```python
from build123d import *

# Parameters (mm, degrees)
EXTRUDE_1_DEPTH       = 244
EXTRUDE_3_DEPTH       = 244
PATTERN_CURVE_1_COUNT = 19
PATTERN_CURVE_1_PITCH = 9.75
SKETCH_3_R            = 2.25
CUT_EXTRUDE_1_DEPTH   = 50
CUT_EXTRUDE_3_DEPTH   = 80
SKETCH_8_R            = 1.6
SKETCH_8_R_2          = 1.3
CUT_EXTRUDE_4_DEPTH   = 10
SKETCH_10_R           = 2.6
SKETCH_10_R_2         = 1.6
CUT_EXTRUDE_5_DEPTH   = 6
SKETCH_12_R           = 2.1
SKETCH_12_R_2         = 1.6
CUT_EXTRUDE_6_DEPTH   = 10


with BuildPart() as part:
    # Эскиз1 → Вытянуть1 (new body)
    with BuildSketch(Plane.XY):
        with BuildLine():
            Line((0, 45), (2.564446908, 45))
            ThreePointArc((2.564446908, 45), (3.247630994, 44.730246195), (3.562232066, 44.066519011))
            Line((3.562232066, 44.066519011), (5.5, 15))
            Line((5.5, 15), (194.5, 15))
            Line((194.5, 15), (196.437767934, 44.066519011))
            ThreePointArc((196.437767934, 44.066519011), (196.752369006, 44.730246195), (197.435553092, 45))
            Line((197.435553092, 45), (200, 45))
            Line((200, 45), (200, 0))
            Line((200, 0), (0, 0))
            Line((0, 0), (0, 45))
        make_face()
    extrude(amount=EXTRUDE_1_DEPTH)

    # Эскиз2 → Вытянуть3 (add)
    with BuildSketch(Plane.XY.offset(244)):
        with BuildLine():
            Line((11.5, 44.5), (10, 15))
            Line((10, 15), (14, 15))
            Line((14, 15), (12.5, 44.5))
            ThreePointArc((12.5, 44.5), (12, 45), (11.5, 44.5))
        make_face()
    extrude_3 = extrude(amount=-EXTRUDE_3_DEPTH)

    # Кривая1: Вытянуть3 ×19
    with Locations(*[(i * PATTERN_CURVE_1_PITCH, 0, 0) for i in range(1, PATTERN_CURVE_1_COUNT)]):
        add(extrude_3)

    # Эскиз3 → Вырез-Вытянуть1 (cut)
    with BuildSketch(Plane.XZ):
        with Locations((4, 236)):
            Circle(SKETCH_3_R)
        with Locations((74, 236)):
            Circle(SKETCH_3_R)
        with Locations(Location((74, 8, 0), (0, 0, 131.810314896))):
            Circle(SKETCH_3_R)
        with Locations(Location((4, 8, 0), (0, 0, 311.810314896))):
            Circle(SKETCH_3_R)
        with Locations((196, 8)):
            Circle(SKETCH_3_R)
        with Locations((126, 8)):
            Circle(SKETCH_3_R)
        with Locations(Location((126, 236, 0), (0, 0, 63.612200039))):
            Circle(SKETCH_3_R)
        with Locations(Location((196, 236, 0), (0, 0, 309.644601439))):
            Circle(SKETCH_3_R)
    extrude(amount=-CUT_EXTRUDE_1_DEPTH, mode=Mode.SUBTRACT)

    # Эскиз6 → Вырез-Вытянуть3 (cut)
    with BuildSketch(Plane.XZ.offset(-6)):
        with BuildLine():
            Line((9, 236), (9, 247.625328498))
            Line((9, 247.625328498), (-6.127764857, 247.625328498))
            Line((-6.127764857, 247.625328498), (-6.127764857, 231))
            Line((-6.127764857, 231), (4, 231))
            ThreePointArc((4, 231), (7.535533906, 232.464466094), (9, 236))
        make_face()
        with BuildLine():
            Line((69, 236), (69, 248.983105869))
            Line((69, 248.983105869), (79, 248.983105869))
            Line((79, 248.983105869), (79, 236))
            ThreePointArc((79, 236), (74, 231), (69, 236))
        make_face()
        with BuildLine():
            Line((121, 248.983105869), (121, 236))
            ThreePointArc((121, 236), (126, 231), (131, 236))
            Line((131, 236), (131, 248.983105869))
            Line((131, 248.983105869), (121, 248.983105869))
        make_face()
        with BuildLine():
            Line((206.127764857, 247.625328498), (191, 247.625328498))
            Line((191, 247.625328498), (191, 236))
            ThreePointArc((191, 236), (192.464466094, 232.464466094), (196, 231))
            Line((196, 231), (206.127764857, 231))
            Line((206.127764857, 231), (206.127764857, 247.625328498))
        make_face()
        with BuildLine():
            Line((191, 8), (191, -3.625328498))
            Line((191, -3.625328498), (206.127764857, -3.625328498))
            Line((206.127764857, -3.625328498), (206.127764857, 13))
            Line((206.127764857, 13), (196, 13))
            ThreePointArc((196, 13), (192.464466094, 11.535533906), (191, 8))
        make_face()
        with BuildLine():
            Line((131, 8), (131, -4.983105869))
            Line((131, -4.983105869), (121, -4.983105869))
            Line((121, -4.983105869), (121, 8))
            ThreePointArc((121, 8), (126, 13), (131, 8))
        make_face()
        with BuildLine():
            Line((79, -4.983105869), (79, 8))
            ThreePointArc((79, 8), (74, 13), (69, 8))
            Line((69, 8), (69, -4.983105869))
            Line((69, -4.983105869), (79, -4.983105869))
        make_face()
        with BuildLine():
            Line((-6.127764857, -3.625328498), (9, -3.625328498))
            Line((9, -3.625328498), (9, 8))
            ThreePointArc((9, 8), (7.535533906, 11.535533906), (4, 13))
            Line((4, 13), (-6.127764857, 13))
            Line((-6.127764857, 13), (-6.127764857, -3.625328498))
        make_face()
    extrude(amount=-CUT_EXTRUDE_3_DEPTH, mode=Mode.SUBTRACT)

    # Эскиз8 → Вырез-Вытянуть4 (cut)
    with BuildSketch(Plane(origin=(133.240090243, 0, 310.149074448), x_dir=(-1, 0, 0), z_dir=(0, -1, 0))):
        with Locations(Location((93.240090243, 92.149074448, 0), (0, 0, 180))):
            Circle(SKETCH_8_R)
        with Locations(Location((93.240090243, 227.149074448, 0), (0, 0, 180))):
            Circle(SKETCH_8_R)
        with Locations(Location((53.490090243, 223.549074448, 0), (0, 0, 180))):
            Circle(SKETCH_8_R)
        with Locations(Location((53.490090243, 139.749074448, 0), (0, 0, 180))):
            Circle(SKETCH_8_R)
        with Locations(Location((56.240090243, 100.649074448, 0), (0, 0, 180))):
            Circle(SKETCH_8_R_2)
        with Locations(Location((113.240090243, 285.149074448, 0), (0, 0, 180))):
            Circle(SKETCH_8_R)
        with Locations(Location((113.240090243, 237.149074448, 0), (0, 0, 180))):
            Circle(SKETCH_8_R)
        with Locations(Location((47.240090243, 237.149074448, 0), (0, 0, 180))):
            Circle(SKETCH_8_R)
        with Locations(Location((47.240090243, 285.149074448, 0), (0, 0, 180))):
            Circle(SKETCH_8_R)
    extrude(amount=-CUT_EXTRUDE_4_DEPTH, mode=Mode.SUBTRACT)

    # Эскиз10 → Вырез-Вытянуть5 (cut)
    with BuildSketch(Plane(origin=(-5.723570629, 0, -26.359021189), x_dir=(1, 0, 0), z_dir=(0, -1, 0))):
        with Locations((139.223570629, 207.359021189)):
            Circle(SKETCH_10_R)
        with Locations((165.723570629, 244.359021189)):
            Circle(SKETCH_10_R_2)
        with Locations((165.723570629, 109.359021189)):
            Circle(SKETCH_10_R_2)
        with Locations((125.473570629, 196.759021189)):
            Circle(SKETCH_10_R_2)
        with Locations((125.473570629, 112.959021189)):
            Circle(SKETCH_10_R_2)
    extrude(amount=-CUT_EXTRUDE_5_DEPTH, mode=Mode.SUBTRACT)

    # Эскиз12 → Вырез-Вытянуть6 (cut)
    with BuildSketch(Plane(origin=(193.647525499, 0, 525.672067887), x_dir=(-1, 0, 0), z_dir=(0, -1, 0))):
        with Locations(Location((10.647525499, 425.672067887, 0), (0, 0, 180))):
            Circle(SKETCH_12_R)
        with Locations((18.647525499, 500.672067887)):
            Circle(SKETCH_12_R_2)
        with Locations((78.647525499, 500.672067887)):
            Circle(SKETCH_12_R_2)
        with Locations(Location((78.647525499, 465.672067887, 0), (0, 0, 180))):
            Circle(SKETCH_12_R_2)
        with Locations(Location((18.647525499, 465.672067887, 0), (0, 0, 180))):
            Circle(SKETCH_12_R_2)
    extrude(amount=-CUT_EXTRUDE_6_DEPTH, mode=Mode.SUBTRACT)


solid = part.part
```
CAD build for the part. Positions are in the model's coordinates, mm. A direction names the side the tool comes from. Round coordinates to 2 decimals unless told otherwise and drop trailing zeros. Use CSV: the item, a comma, the result in double quotes. Start each with the question number.
1) Pin check, flat tips, straight feed: pin 1 Ø1.7 at (x, z) = (76, 87) entering from +Y; pin 2 Ø1 at (x, y) = (126.5, 33) entering from +Z; pin 3 Ø5 at (x, z) = (122.5, 62.5) entering from -Y; pin 4 Ø1.6 at (x, z) = (20.5, 25.5) entering from -Y. Stop position of each tip, or through.
2) Two-plate mould, pull along X, no slides. Class faces 3 (the cylindrical face through (7, 11, 12)), 4 (the flat face through (195, 6, 239)), 5 (the flat face through (188.76, 29.54, 123.71)): pulls with the +X half, pulls with the -X half, needs draft (parallel to the pull), parting line crosses it, or undercut.
3) Tool access for faces 1 (the flat face through (163, 15, 120)), 2 (the flat face through (69, 15, 240)): list every direction of +Z, -Z, +X, -X, +Y, -Y with a clear straight run to the whole face (end or side of a thin tool).
4) Wall check: L1, parallel to Z at x = 4, y = 3; L2, parallel to Z at x = 79.75, y = 6.75; L3, parallel to X at y = 3.6, z = 236. Give the ranges that are in metal, low to high. Write a range as [from, to].
Values follow:
1,pin 1,"stops at y = 15"
1,pin 2,"passes through"
1,pin 3,"stops at y = 0"
1,pin 4,"stops at y = 10"
2,face 3,"pulls with the -X half"
2,face 4,"needs draft"
2,face 5,"undercut"
3,face 1,"+Z, -Z, +Y"
3,face 2,"+Z, +Y"
4,L1,"z = [0, 5.75], [10.25, 233.75], [238.25, 244]"
4,L2,"z = [0, 85], [88.2, 168.8], [172, 244]"
4,L3,"x = [0, 1.75], [6.25, 71.75], [76.25, 123.75], [128.25, 193.75], [198.25, 200]"
